```python
from build123d import *

# Parameters (mm, degrees)
SKETCH1_W            = 48
SKETCH1_H            = 50
BOSS_EXTRUDE1_DEPTH  = 39
M6_CLEARANCE_HOLE1_D = 6.6
CUT_EXTRUDE1_DEPTH   = 80.529868603


with BuildPart() as part:
    # Sketch1 → Boss-Extrude1 (new body)
    with BuildSketch(Plane(origin=(0, 0, 0), x_dir=(1, 0, 0), z_dir=(0, 1, 0))):
        with Locations((24, 25)):
            Rectangle(SKETCH1_W, SKETCH1_H)
    extrude(amount=BOSS_EXTRUDE1_DEPTH)

    # M6 Clearance Hole1 (through all)
    with Locations(Plane(origin=(0, 39, 0), x_dir=(1, 0, 0), z_dir=(0, 1, 0))):
        with Locations((6.5, 42.5), (41.5, 42.5), (41.5, 7.5), (6.5, 7.5), (24, 25)):
            Hole(M6_CLEARANCE_HOLE1_D / 2)

    # Sketch4 → Cut-Extrude1 (cut, through all)
    with BuildSketch(Plane.XY):
        with BuildLine():
            Line((30.25, 2.364109857), (31.614919462, 0))
            Line((31.614919462, 0), (16.385080538, 0))
            Line((16.385080538, 0), (17.75, 2.364109857))
            ThreePointArc((17.75, 2.364109857), (24, 31), (30.25, 2.364109857))
        make_face()
    extrude(amount=-CUT_EXTRUDE1_DEPTH, mode=Mode.SUBTRACT)


solid = part.part
```
Part model, mm, in its own coordinate system. A direction names the side the tool comes from. Round coordinates to 2 decimals unless told otherwise and drop trailing zeros. Loops run counter-clockwise (first coordinate to the right, second up) from the corner with the lowest first, then second, coordinate; pieces in that order, holes last. Notation, with made-up numbers: (68, 51.25) -> (85, 51.25) arc R25 cw to (85, 73.25) -> close; hole circle Ø8 at (70, -30). An arc over 180 degrees is marked (long way). Use one line per item in the form item = value. Start each with the question number.
Item 1: Band-saw the part on D-D (z = -13.5). List the corners of the cut face in (x, y).
Item 2: Tool access for faces 1 (the flat face through (30.92, 1.2, -24.65)), 2 (the cylindrical face through (32.03, 28.67, -24.65)): list every direction of +Z, -Z, +X, -X, +Y, -Y with a clear straight run to the whole face (end or side of a thin tool).
Item 3: Band-saw the part on A-A (y = 7). List the corners of the cut face in (x, z), plus the area to 3 significant figures.
Item 4: Drop flat-ended pins along their axis: pin 1 Ø7.5 at (x, z) = (24, -25) entering from -Y; pin 2 Ø1 at (x, z) = (18.5, -28) entering from -Y; pin 3 Ø4 at (x, z) = (6.5, -42.5) entering from +Y. Give the stop position or say it passes through.
Item 5: Two-plate mould, pull along Z, no slides. Class faces 3 (the flat face through (24, 32, -50)), 4 (the flat face through (17.06, 1.17, -24.65)), 5 (the cylindrical face through (44.8, 19.2, -7.6)): released by +Z, released by -Z, zero draft, split by the parting line, or undercut.
Item 6: Band-saw the part on B-B (x = 24). List the corners of the cut face in (y, z).
Item 7: Band-saw the part on C-C (x = 6.5). List the corners of the cut face in (y, z).
Item 8: Drill centre lines: line 1 along Z through (x, y) = (6.5, 14.5); line 2 along X through (y, z) = (16, -25); line 3 along Y through (x, z) = (24, -10). Where is each one in solid material? Low to high.
Data:
q1.outline = (0, 0) -> (16.39, 0) -> (17.75, 2.36) arc R15 cw (long way) to (30.25, 2.36) -> (31.61, 0) -> (48, 0) -> (48, 39) -> (0, 39) -> close
q2.face_1 = +Z, -Z, -Y
q2.face_2 = +Z, -Z
q3.outline = (0, -50) -> (12, -50) -> (12, 0) -> (0, 0) -> close; (36, -50) -> (48, -50) -> (48, 0) -> (36, 0) -> close; hole circle Ø6.6 at (6.5, -42.5); hole circle Ø6.6 at (6.5, -7.5); hole circle Ø6.6 at (41.5, -42.5); hole circle Ø6.6 at (41.5, -7.5)
q3.area = 1,060 mm^2
q4.pin_1 = 30.52
q4.pin_2 = 29.75
q4.pin_3 = through
q5.face_3 = released by -Z
q5.face_4 = zero draft
q5.face_5 = undercut
q6.outline = (31, -50) -> (39, -50) -> (39, -28.3) -> (31, -28.3) -> close; (31, -21.7) -> (39, -21.7) -> (39, 0) -> (31, 0) -> close
q7.outline = (0, -50) -> (39, -50) -> (39, -45.8) -> (0, -45.8) -> close; (0, -39.2) -> (39, -39.2) -> (39, -10.8) -> (0, -10.8) -> close; (0, -4.2) -> (39, -4.2) -> (39, 0) -> (0, 0) -> close
q8.line_1 = -50 to -45.8, -39.2 to -10.8, -4.2 to 0
q8.line_2 = 0 to 9, 39 to 48
q8.line_3 = 31 to 39
